from build123d import *

# Parameters (mm, degrees)
SKETCH1_R           = 2
BOSS_EXTRUDE1_DEPTH = 2
FILLET1_R           = 10


with BuildPart() as part:
    # Sketch1 → Boss-Extrude1 (new body)
    with BuildSketch(Plane(origin=(0, 0, 0), x_dir=(1, 0, 0), z_dir=(0, 1, 0))):
        Polygon((50, 12.5), (50, -12.5), (15, -12.5), (15, -17.5), (-15, -17.5), (-15, -12.5), (-50, -12.5), (-50, 12.5), align=None)
        with Locations(Location((-9, -13.5, 0), (0, 0, 270))):
            Circle(SKETCH1_R, mode=Mode.SUBTRACT)
        with Locations(Location((9, -13.5, 0), (0, 0, 270))):
            Circle(SKETCH1_R, mode=Mode.SUBTRACT)
    extrude(amount=BOSS_EXTRUDE1_DEPTH)

    # Fillet1
    fillet1_edges = [part.edges().sort_by_distance(p)[0] for p in [
        (-50, 1, -12.5),
        (50, 1, -12.5),
    ]]
    fillet(fillet1_edges, radius=FILLET1_R)


solid = part.part
Work out the finished part from the listing and answer in its coordinate system (mm). A direction names the side the tool comes from. Give positions to 0.01 mm unless a question says otherwise; leave off trailing zeros. Loops run counter-clockwise (first coordinate to the right, second up) from the corner with the lowest first, then second, coordinate; pieces in that order, holes last. Notation, with made-up numbers: (-38.75, 16.5) - (-32.75, 16.5) arc R19 ccw to (-32.75, 39.5) - close; hole circle Ø6 at (81.25, -31.5). An arc over 180 degrees is marked (long way). Answer in a Markdown table with one row per item. Add a question column.
Q1. The part is cut by section B-B (y = 1.1). Determine the outline of the cut face in (x, z).
Q2. Consider line 1 along X through (y, z) = (0.6, 13.5); line 2 along Z through (x, y) = (34, 1.95); line 3 along X through (y, z) = (1.2, 13). Determine where each line is inside the solid, lowest interval first.
Q3. The part is cut by section C-C (x = 9). Determine the outline of the cut face in (y, z).
Q4. Determine the mould class of faces 4 (the flat face through (0, 1, 17.5)), 5 (the cylindrical face through (10.352, 0.986, 12.026)), 6 (the flat face through (-50, 1, 5)) for opening direction Z: released by +Z, released by -Z, zero draft, split by the parting line, or undercut.
Q5. The part is cut by section D-D (x = -37). Determine the outline of the cut face in (y, z).
Q6. Each of these flat-tipped pins is pushed along its axis until it touches: P1, Ø1, axis at x = -25.5, y = 0.5, coming from the +Z side; P2, Ø0.6, axis at y = 1.5, z = 14.5, coming from the -X side. Where does it stop, or does it pass through?
Q7. A tool of negligible diameter and unlimited length cuts with its end or side. For faces 1 (the flat face through (33, 1, 12.5)), 2 (the flat face through (-15, 1, 15)), 3 (the flat face through (50, 1, 5)), from which of +Z, -Z, +X, -X, +Y, -Y can it reach the whole face along a straight path? Write none if from no direction.
Q8. The part is cut by section A-A (z = 13.5). Determine the outline of the cut face in (x, y), and give its area (3 significant figures).
Solution:
| question | item | result |
|---|---|---|
| 1 | outline | (-50, -2.5) arc R10 ccw to (-40, -12.5) - (40, -12.5) arc R10 ccw to (50, -2.5) - (50, 12.5) - (15, 12.5) - (15, 17.5) - (-15, 17.5) - (-15, 12.5) - (-50, 12.5) - close; hole circle Ø4 at (-9, 13.5); hole circle Ø4 at (9, 13.5) |
| 2 | line 1 | x = -15 to -11, -7 to 7, 11 to 15 |
| 2 | line 2 | z = -12.5 to 12.5 |
| 2 | line 3 | x = -15 to -10.94, -7.06 to 7.06, 10.94 to 15 |
| 3 | outline | (0, -12.5) - (2, -12.5) - (2, 11.5) - (0, 11.5) - close; (0, 15.5) - (2, 15.5) - (2, 17.5) - (0, 17.5) - close |
| 4 | face 4 | released by +Z |
| 4 | face 5 | undercut |
| 4 | face 6 | zero draft |
| 5 | outline | (0, -12.5) - (2, -12.5) - (2, 12.5) - (0, 12.5) - close |
| 6 | P1 | stops at z = 12.5 |
| 6 | P2 | stops at x = -15 |
| 7 | face 1 | +Z, +X, +Y, -Y |
| 7 | face 2 | +Z, -X, +Y, -Y |
| 7 | face 3 | +Z, -Z, +X, +Y, -Y |
| 8 | outline | (-15, 0) - (-11, 0) - (-11, 2) - (-15, 2) - close; (-7, 0) - (7, 0) - (7, 2) - (-7, 2) - close; (11, 0) - (15, 0) - (15, 2) - (11, 2) - close |
| 8 | area | 44.0 mm² |
